Could you check a few things on this model? Use its own coordinates, in mm. A direction names the side the tool comes from. Round coordinates to 2 decimals unless told otherwise and drop trailing zeros. Order: outer loops, then holes, each group sorted by start corner. A loop starts at its lowest first (then second) coordinate and runs counter-clockwise, first axis right, second up. Notation, with made-up numbers: M 2,17 L 33,17 A8 ccw 33,26 Z; hole C 27,-2 d11. An arc over 180 degrees is marked long. Write each question's results on one line, items separated by ' | '. Start each with the question number.
1. I'm going to push flat-ended pins straight in: pin 1 (6 mm diameter, centred on x = -14, z = -10.5, fed in from +Y); pin 2 (10 mm diameter, centred on x = -27.5, z = -4.5, fed in from +Y); pin 3 (3.5 mm diameter, centred on y = 33, z = 0, fed in from +X). Where does each tip first touch, or does it pass through?
2. Suppose I cut it at A-A on z = -20. Write out the boundary of the cut face in (x, y), and give its area (3 significant figures).
3. We'd pull the mould along Z, two halves only. Please class faces 1 (the flat face through (-1, 70, -40)), 2 (the flat face through (0, -20, -6)), 3 (the cylindrical face through (-18.6, -22.5, 17.9)): released by +Z, released by -Z, zero draft, split by the parting line, or undercut.
4. Please list where these lines run through material, in increasing order: L1, parallel to Z at x = 13, y = 41; L2, parallel to X at y = 42, z = 14; L3, parallel to Y at x = -1.5, z = -31.
5. For faces 4 (the flat face through (35.1, 22, -40)), 5 (the flat face through (-20, 28, -8)), 6 (the flat face through (15, 30, -10)), 7 (the flat face through (0, 55, -22)), which set-ups out of +Z, -Z, +X, -X, +Y, -Y let a thin tool reach every point of the face, with its end or its side?
6. Suppose I cut it at C-C on y = -8.5. Write out the boundary of the cut face in (x, z), and give its area (3 significant figures).
7. Suppose I cut it at D-D on z = 0.4. Write out the boundary of the cut face in (x, y), and give its area (3 significant figures).
8. Suppose I cut it at B-B on x = 7. Write out the boundary of the cut face in (y, z).
from build123d import *

# Parameters (mm, degrees)
SKETCH_1_W           = 40
SKETCH_1_H           = 60
EXTRUDE_1_DEPTH      = 55
CUT_EXTRUDE_1_DEPTH  = 50
SKETCH_6_W           = 50
SKETCH_6_H           = 70
EXTRUDE_2_DEPTH      = 25
SKETCH_7_W           = 60
SKETCH_7_H           = 15
CUT_EXTRUDE_2_DEPTH  = 51
CUT_EXTRUDE_3_REACH  = 82
SKETCH_10_W          = 80
SKETCH_10_H          = 5
EXTRUDE_3_DEPTH      = 70
EXTRUDE_3_DEPTH_BACK = 25
CUT_EXTRUDE_4_REACH  = 72
FILLET_1_R           = 2
FILLET_2_R           = 1
FILLET_3_R           = 1


with BuildPart() as part:
    # 草图1 → 凸台-拉伸1 (new body)
    with BuildSketch(Plane(origin=(0, 0, 0), x_dir=(1, 0, 0), z_dir=(0, 1, 0))):
        with Locations((0, 10)):
            Rectangle(SKETCH_1_W, SKETCH_1_H)
    extrude(amount=EXTRUDE_1_DEPTH)

    # 草图2 → 切除-拉伸1 (cut)
    with BuildSketch(Plane(origin=(0, 55, 0), x_dir=(1, 0, 0), z_dir=(0, 1, 0))):
        Polygon((-15, 15), (-15, 3.1), (-11, 3.1), (-11, -4), (-15, -4), (-15, -15), (15, -15), (15, -4), (11, -4), (11, 3.1), (15, 3.1), (15, 15), (15, 18), (-15, 18), align=None)
    extrude(amount=-CUT_EXTRUDE_1_DEPTH, mode=Mode.SUBTRACT)

    # 草图6 → 凸台-拉伸2 (add)
    with BuildSketch(Plane(origin=(0, 0, 0), x_dir=(-1, 0, 0), z_dir=(0, -1, 0))):
        with Locations((0, 7)):
            Rectangle(SKETCH_6_W, SKETCH_6_H)
    extrude(amount=EXTRUDE_2_DEPTH)

    # 草图7 → 切除-拉伸2 (cut, through all)
    with BuildSketch(Plane(origin=(25, 0, 0), x_dir=(0, 0, -1), z_dir=(1, 0, 0))):
        with Locations((7, -12.5)):
            Rectangle(SKETCH_7_W, SKETCH_7_H)
    extrude(amount=-CUT_EXTRUDE_2_DEPTH, mode=Mode.SUBTRACT)

    # 草图8 → 切除-拉伸3 (cut, up to next)
    with BuildSketch(Plane.XZ.offset(25), mode=Mode.PRIVATE) as cut_extrude_3_sk1:
        with BuildLine():
            Line((-16, 20.6), (16, 20.6))
            ThreePointArc((16, 20.6), (18.6, 18), (16, 15.4))
            Line((16, 15.4), (-16, 15.4))
            ThreePointArc((-16, 15.4), (-18.6, 18), (-16, 20.6))
        make_face()
    cut_extrude_3_tool1 = extrude(cut_extrude_3_sk1.sketch, amount=-CUT_EXTRUDE_3_REACH, mode=Mode.PRIVATE) & part.part
    add(cut_extrude_3_tool1.solids().sort_by_distance((0, -25, 18))[0], mode=Mode.SUBTRACT)
    # 草图8 → 切除-拉伸3 (cut, up to next)
    with BuildSketch(Plane.XZ.offset(25), mode=Mode.PRIVATE) as cut_extrude_3_sk2:
        with BuildLine():
            Line((-16, 3), (16, 3))
            ThreePointArc((16, 3), (18.6, 0.4), (16, -2.2))
            Line((16, -2.2), (-16, -2.2))
            ThreePointArc((-16, -2.2), (-18.6, 0.4), (-16, 3))
        make_face()
    cut_extrude_3_tool2 = extrude(cut_extrude_3_sk2.sketch, amount=-CUT_EXTRUDE_3_REACH, mode=Mode.PRIVATE) & part.part
    add(cut_extrude_3_tool2.solids().sort_by_distance((0, -25, 0.4))[0], mode=Mode.SUBTRACT)

    # 草图10 → 凸台-拉伸3 (add, two sides)
    with BuildSketch(Plane(origin=(0, 0, 0), x_dir=(1, 0, 0), z_dir=(0, 1, 0))) as extrude_3_sk:
        with Locations((0, 39.5)):
            Rectangle(SKETCH_10_W, SKETCH_10_H)
    extrude(amount=EXTRUDE_3_DEPTH)
    extrude(extrude_3_sk.sketch, amount=-EXTRUDE_3_DEPTH_BACK)

    # 草图11 → 切除-拉伸4 (cut, up to next)
    with BuildSketch(Plane(origin=(0, 0, -42), x_dir=(-1, 0, 0), z_dir=(0, 0, -1)), mode=Mode.PRIVATE) as cut_extrude_4_sk1:
        with BuildLine():
            Line((-29.9, 62), (-29.9, -17))
            ThreePointArc((-29.9, -17), (-32.5, -19.6), (-35.1, -17))
            Line((-35.1, -17), (-35.1, 62))
            ThreePointArc((-35.1, 62), (-32.5, 64.6), (-29.9, 62))
        make_face()
    cut_extrude_4_tool1 = extrude(cut_extrude_4_sk1.sketch, amount=-CUT_EXTRUDE_4_REACH, mode=Mode.PRIVATE) & part.part
    add(cut_extrude_4_tool1.solids().sort_by_distance((32.5, 22.5, -42))[0], mode=Mode.SUBTRACT)
    # 草图11 → 切除-拉伸4 (cut, up to next)
    with BuildSketch(Plane(origin=(0, 0, -42), x_dir=(-1, 0, 0), z_dir=(0, 0, -1)), mode=Mode.PRIVATE) as cut_extrude_4_sk2:
        with BuildLine():
            Line((29.9, 62), (29.9, -17))
            ThreePointArc((29.9, -17), (32.5, -19.6), (35.1, -17))
            Line((35.1, -17), (35.1, 62))
            ThreePointArc((35.1, 62), (32.5, 64.6), (29.9, 62))
        make_face()
    cut_extrude_4_tool2 = extrude(cut_extrude_4_sk2.sketch, amount=-CUT_EXTRUDE_4_REACH, mode=Mode.PRIVATE) & part.part
    add(cut_extrude_4_tool2.solids().sort_by_distance((-32.5, 22.5, -42))[0], mode=Mode.SUBTRACT)

    # 圆角1
    fillet_1_edges = [part.edges().sort_by_distance(p)[0] for p in [
        (-40, 22.5, -42),
        (40, 22.5, -37),
        (20, 27.5, -37),
        (-20, 27.5, -37),
        (-40, 22.5, -37),
        (-40, -25, -39.5),
        (40, 22.5, -42),
        (40, -25, -39.5),
        (-40, 70, -39.5),
        (40, 70, -39.5),
        (0, 0, 28),
        (25, -12.5, 28),
        (-25, -12.5, 28),
        (0, -25, 28),
        (20, 27.5, 20),
        (-20, 27.5, 20),
    ]]
    fillet(fillet_1_edges, radius=FILLET_1_R)

    # 圆角2
    fillet_2_edges = [part.edges().sort_by_distance(p)[0] for p in [
        (-23.5, 0, -37),
        (23.5, 0, -37),
        (20, 0, -8.5),
        (0, 0, 20),
        (-20, 0, -8.5),
        (-20.585786438, 0, -36.414213562),
        (20.585786438, 0, -36.414213562),
        (19.414213562, 0, 19.414213562),
        (-19.414213562, 0, 19.414213562),
    ]]
    fillet(fillet_2_edges, radius=FILLET_2_R)

    # 圆角3
    fillet_3_edges = [part.edges().sort_by_distance(p)[0] for p in [
        (25, -12.5, 23),
        (-25, -12.5, 23),
        (-25, -22.5, -37),
        (-25, -2.5, -37),
        (25, -22.5, -37),
        (25, -2.5, -37),
    ]]
    fillet(fillet_3_edges, radius=FILLET_3_R)


solid = part.part
Filled sheet:
1) pin 1: stops at y = 55 | pin 2: stops at y = 0 | pin 3: stops at x = 20
2) outline: M -25,-25 L 25,-25 L 25,-20 L -25,-20 Z; M -25,-5 L 25,-5 L 25,0 L 21,0 A1 cw 20,1 L 20,55 L -20,55 L -20,1 A1 cw -21,0 L -25,0 Z | area: 2,700 mm^2
3) face 1: zero draft | face 2: undercut | face 3: undercut
4) L1: z = -42 to -18, -3.1 to 4, 15 to 20 | L2: x = -20 to -15, 15 to 20 | L3: y = -25 to -20, -5 to 55
5) face 4: +Z, -Z | face 5: +Z, -X, +Y | face 6: +Y | face 7: +Z, +X, -X, +Y
6) outline: M -40,-40 A2 ccw -38,-42 L -35.1,-42 L -35.1,-37 L -38,-37 A2 ccw -40,-39 Z; M -29.9,-42 L 29.9,-42 L 29.9,-37 L -29.9,-37 Z; M -25,24 A1 ccw -24,23 L 24,23 A1 ccw 25,24 L 25,26 A2 ccw 23,28 L -23,28 A2 ccw -25,26 Z; M 35.1,-42 L 38,-42 A2 ccw 40,-40 L 40,-39 A2 ccw 38,-37 L 35.1,-37 Z | area: 592 mm^2
7) outline: M -25,-25 L -18.6,-25 L -18.6,-20 L -25,-20 Z; M -25,-5 L 25,-5 L 25,0 L 21,0 A1 cw 20,1 L 20,55 L 11,55 L 11,5 L -11,5 L -11,55 L -20,55 L -20,1 A1 cw -21,0 L -25,0 Z; M 18.6,-25 L 25,-25 L 25,-20 L 18.6,-20 Z | area: 1,410 mm^2
8) outline: M -25,-42 L 70,-42 L 70,-37 L 55,-37 L 55,-18 L 5,-18 L 5,15 L 55,15 L 55,20 L 1,20 A1 cw 0,21 L 0,26 A2 ccw -2,28 L -23,28 A2 ccw -25,26 L -25,20.6 L -20,20.6 L -20,23 L -5,23 L -5,-37 L -20,-37 L -20,-2.2 L -25,-2.2 Z; M -25,3 L -20,3 L -20,15.4 L -25,15.4 Z
